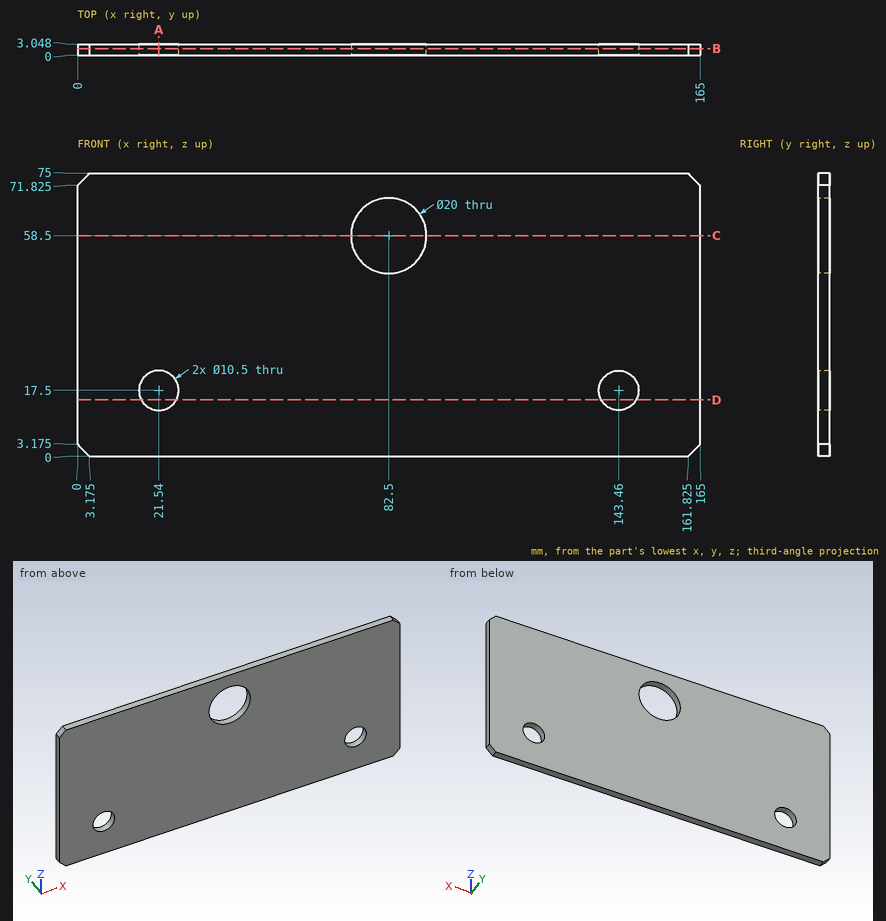
Geometry check sheet. Reference: drawing and pictorial views, mm from the part's lowest x, y, z. Coordinates: 2 decimals unless noted, no trailing zeros. Write each loop counter-clockwise with the first axis right and the second up, starting at its lowest first coordinate (ties: lowest second). Pieces come first, ordered by that corner, then holes. Notation, with made-up numbers: (10.5, 20.25) -> (53.5, 20.25) arc R15 cw to (53.5, 39.25) -> close; hole circle Ø10 at (72.5, 89.5). An arc over 180 degrees is marked (long way). Use a Markdown table: item, result.
1. Sectioned sample at A-A (x = 21.54). Enter the section's corners in (y, z), plus the area to 3 significant figures.
Reported:
| item | result |
|---|---|
| outline | (0, 0) -> (3.05, 0) -> (3.05, 12.25) -> (0, 12.25) -> close; (0, 22.75) -> (3.05, 22.75) -> (3.05, 75) -> (0, 75) -> close |
| area | 197 mm2 |
2. Sectioned sample at D-D (z = 15). Enter the section's corners in (x, y).
Reported:
| item | result |
|---|---|
| outline | (0, 0) -> (16.92, 0) -> (16.92, 3.05) -> (0, 3.05) -> close; (26.16, 0) -> (138.84, 0) -> (138.84, 3.05) -> (26.16, 3.05) -> close; (148.08, 0) -> (165, 0) -> (165, 3.05) -> (148.08, 3.05) -> close |
3. Scan lines: line 1 along Z through (x, y) = (82.5, 1.55); line 2 along Z through (x, y) = (143.46, 1.6); line 3 along X through (y, z) = (2.8, 62.5). Record each from-to range of solid material in increasing order.
Reported:
| item | result |
|---|---|
| line 1 | z = 0 to 48.5, 68.5 to 75 |
| line 2 | z = 0 to 12.25, 22.75 to 75 |
| line 3 | x = 0 to 73.33, 91.67 to 165 |
4. Go/stop test with a flat-tipped pin: pin 1 Ø17 at (x, z) = (21.54, 17.5) entering from +Y. Record where the tip stops, or that it passes through.
Reported:
| item | result |
|---|---|
| pin 1 | stops at y = 3.05 |
5. Sectioned sample at C-C (z = 58.5). Enter the section's corners in (x, y).
Reported:
| item | result |
|---|---|
| outline | (0, 0) -> (72.5, 0) -> (72.5, 3.05) -> (0, 3.05) -> close; (92.5, 0) -> (165, 0) -> (165, 3.05) -> (92.5, 3.05) -> close |
6. Sectioned sample at B-B (y = 1.85). Enter the section's corners in (x, z) (3 decimals), plus the area to 3 significant figures.
Reported:
| item | result |
|---|---|
| outline | (0, 3.175) -> (3.175, 0) -> (161.825, 0) -> (165, 3.175) -> (165, 71.825) -> (161.825, 75) -> (3.175, 75) -> (0, 71.825) -> close; hole circle Ø10.5 at (21.54, 17.5); hole circle Ø20 at (82.5, 58.5); hole circle Ø10.5 at (143.46, 17.5) |
| area | 11,900 mm2 |
